```python
from build123d import *

# Parameters (mm, degrees)
SKETCH1_W               = 27.54
SKETCH1_H               = 6.8
BOSS_EXTRUDE1_DEPTH     = 8
SKETCH4_W               = 27.54
SKETCH4_H               = 6.8
BOSS_EXTRUDE2_DEPTH     = 6
CUT_EXTRUDE2_DEPTH      = 18.316261144
CUT_EXTRUDE2_DEPTH_BACK = 18.316261144
SKETCH3_R               = 1.65
SKETCH7_W               = 8
SKETCH7_H               = 20
BOSS_EXTRUDE3_DEPTH     = 6.8
FILLET1_R               = 2


with BuildPart() as part:
    # Sketch1 → Boss-Extrude1 (new body)
    with BuildSketch(Plane.XY):
        Rectangle(SKETCH1_W, SKETCH1_H)
    extrude(amount=BOSS_EXTRUDE1_DEPTH)

    # Sketch4 → Boss-Extrude2 (add)
    with BuildSketch(Plane(origin=(0, 0, 0), x_dir=(-1, 0, 0), z_dir=(0, 0, -1))):
        Rectangle(SKETCH4_W, SKETCH4_H)
    extrude(amount=BOSS_EXTRUDE2_DEPTH)

    # Sketch3 → Cut-Extrude2 (cut, two sides: drawn at the far end of the back side and taken through both)
    with BuildSketch(Plane.XZ.offset(3.4).offset(-CUT_EXTRUDE2_DEPTH_BACK)):
        with Locations(Location((8.73, -3, 0), (0, 0, 270))):
            Circle(SKETCH3_R)
        with Locations(Location((-10.27, -3, 0), (0, 0, 270))):
            Circle(SKETCH3_R)
    extrude(amount=CUT_EXTRUDE2_DEPTH + CUT_EXTRUDE2_DEPTH_BACK, mode=Mode.SUBTRACT)

    # Sketch7 → Boss-Extrude3 (add)
    with BuildSketch(Plane(origin=(0, 3.4, 0), x_dir=(1, 0, 0), z_dir=(0, 1, 0))):
        with Locations((-17.77, -4)):
            Rectangle(SKETCH7_W, SKETCH7_H)
        with BuildLine():
            Line((-16.12, 3), (-16.12, 0))
            ThreePointArc((-16.12, 0), (-17.77, -1.65), (-19.42, 0))
            Line((-19.42, 0), (-19.42, 3))
            ThreePointArc((-19.42, 3), (-17.77, 4.65), (-16.12, 3))
        make_face(mode=Mode.SUBTRACT)
        with BuildLine():
            Line((-16.12, -7), (-16.12, -10))
            ThreePointArc((-16.12, -10), (-17.77, -11.65), (-19.42, -10))
            Line((-19.42, -10), (-19.42, -7))
            ThreePointArc((-19.42, -7), (-17.77, -5.35), (-16.12, -7))
        make_face(mode=Mode.SUBTRACT)
    extrude(amount=-BOSS_EXTRUDE3_DEPTH)

    # Fillet1
    fillet1_edges = [part.edges().sort_by_distance(p)[0] for p in [
        (13.77, 0, -6),
        (-13.77, 0, 8),
        (-21.77, 0, -6),
        (-21.77, 0, 14),
        (-13.77, 0, 14),
        (13.77, 0, 8),
    ]]
    fillet(fillet1_edges, radius=FILLET1_R)


solid = part.part
```
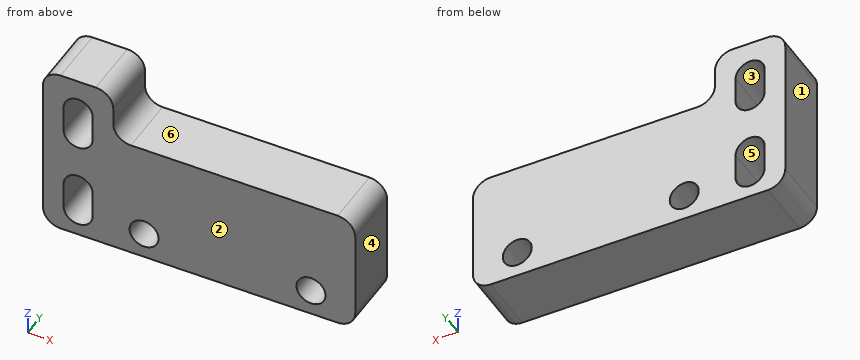
Work out the finished part from the listing and answer in its coordinate system (mm). Face numbers are marked on the shaded views. A direction names the side the tool comes from. Round coordinates to 2 decimals unless told otherwise and drop trailing zeros. Loops run counter-clockwise (first coordinate to the right, second up) from the corner with the lowest first, then second, coordinate; pieces in that order, holes last. Notation, with made-up numbers: M -34,44.25 L -25,44.25 A13 ccw -25,63.25 Z; hole C 9,-24 d9. An arc over 180 degrees is marked long. Use CSV: the item, a comma, the result in double quotes.
Q1. Section A-A, the plane y = -2 is taken. Determine the outline of the cut face in (x, z), then the cut area to 3 significant figures.
Determined:
outline,"M -21.77,-4 A2 ccw -19.77,-6 L 11.77,-6 A2 ccw 13.77,-4 L 13.77,6 A2 ccw 11.77,8 L -11.77,8 A2 cw -13.77,10 L -13.77,12 A2 ccw -15.77,14 L -19.77,14 A2 ccw -21.77,12 Z; hole M -19.42,-3 A1.65 ccw -16.12,-3 L -16.12,0 A1.65 ccw -19.42,0 Z; hole M -19.42,7 A1.65 ccw -16.12,7 L -16.12,10 A1.65 ccw -19.42,10 Z; hole C -10.27,-3 d3.3; hole C 8.73,-3 d3.3"
area,"488 mm2"
Q2. A tool of negligible diameter and unlimited length cuts with its end or side. For the marked faces 4, 5 and 6, from which of +Z, -Z, +X, -X, +Y, -Y can it reach the whole face along a straight path? Write none if from no direction.
Determined:
face 4,"+Z, -Z, +X, +Y, -Y"
face 5,"+Y, -Y"
face 6,"+Z, +X, +Y, -Y"
Q3. Section C-C, the plane z = -2 is taken. Determine the outline of the cut face in (x, y), then the cut area to 3 significant figures.
Determined:
outline,"M -21.77,-3.4 L -19.42,-3.4 L -19.42,3.4 L -21.77,3.4 Z; M -16.12,-3.4 L -11.58,-3.4 L -11.58,3.4 L -16.12,3.4 Z; M -8.96,-3.4 L 7.42,-3.4 L 7.42,3.4 L -8.96,3.4 Z; M 10.04,-3.4 L 13.77,-3.4 L 13.77,3.4 L 10.04,3.4 Z"
area,"184 mm2"
Q4. The mould has two halves that part along X. Classify the marked faces 1, 2 and 3: pulls with the +X half, pulls with the -X half, needs draft (parallel to the pull), parting line crosses it, or undercut.
Determined:
face 1,"pulls with the -X half"
face 2,"needs draft"
face 3,"undercut"
Q5. Consider L1, parallel to X at y = 0.75, z = -3; L2, parallel to Z at x = 8.73, y = 1.5; L3, parallel to X at y = -2, z = -0.5. Determine where each line is inside the solid, lowest interval first.
Determined:
L1,"-21.77 to -19.42, -16.12 to -11.92, -8.62 to 7.08, 10.38 to 13.77"
L2,"-6 to -4.65, -1.35 to 8"
L3,"-21.77 to -19.42, -16.12 to 13.77"
Q6. Section B-B, the plane x = 8.73 is taken. Determine the outline of the cut face in (y, z).
Determined:
outline,"M -3.4,-6 L 3.4,-6 L 3.4,-4.65 L -3.4,-4.65 Z; M -3.4,-1.35 L 3.4,-1.35 L 3.4,8 L -3.4,8 Z"
Q7. Each of these flat-tipped pins is pushed along its axis until it touches: pin 1 (2 mm diameter, centred on x = 0.5, y = -1.5, fed in from +Z); pin 2 (1.5 mm diameter, centred on y = 1.5, z = 8.5, fed in from +X); pin 3 (2 mm diameter, centred on y = 1, z = 11, fed in from +X). Where does it stop, or does it pass through?
Determined:
pin 1,"z = 8"
pin 2,"x = 12.74"
pin 3,"x = -13.77"
Q8. Section D-D, the plane x = -17.77 is taken. Determine the outline of the cut face in (y, z).
Determined:
outline,"M -3.4,-6 L 3.4,-6 L 3.4,-4.65 L -3.4,-4.65 Z; M -3.4,1.65 L 3.4,1.65 L 3.4,5.35 L -3.4,5.35 Z; M -3.4,11.65 L 3.4,11.65 L 3.4,14 L -3.4,14 Z"
